Autodesk Inventor part; units mm, degrees
ref_plane "YZ Plane" through (0, 0, 0) normal (1, 0, 0) x (0, 1, 0)
ref_plane "XZ Plane" through (0, 0, 0) normal (0, 1, 0) x (-1, 0, 0)
ref_plane "XY Plane" through (0, 0, 0) normal (0, 0, 1) x (1, 0, 0)
sketch "Sketch1" plane through (0, 0, 0) normal (0, 1, 0) x (-1, 0, 0)
  line L0 (0, -2) -> (0, -29.2)
  line L1 (-2, -31.2) -> (-39, -31.2)
  line L2 (-39, -31.2) -> (-39, -20.2)
  line L3 (-39, -20.2) -> (-37, -20.2)
  line L4 (-37, -20.2) -> (-37, -10.9)
  line L5 (-37, -10.9) -> (-39, -10.9)
  line L6 (-39, -10.9) -> (-39, -2.6)
  line L7 (-39, -2.6) -> (-32.7, -2.6)
  line L8 (-32.7, -2.6) -> (-32.7, 0)
  line L9 (-32.7, 0) -> (-2, 0)
  line L10 (0, -2) -> (-2, 0)
  line L11 (0, -29.2) -> (-2, -31.2)
  point P0 (0, 0)
  point P1 (0, -31.2)
  dimension "d0" = 31.2
  dimension "d1" = 39
  dimension "d2" = 11
  dimension "d3" = 2
  dimension "d4" = 9.3
  dimension "d5" = 8.3
  dimension "d6" = 6.3
  dimension "d7" = 2
  dimension "d8" = 2
  dimension "d9" = 2
  dimension "d10" = 2
extrude "Extrusion1" add sketch "Sketch1" along normal blind 1
sketch "Sketch2" plane through (0, 1, 0) normal (0, 1, 0) x (1, 0, 0)
  line L0 (39, 31.2) -> (2, 31.2)
  line L1 (2, 31.2) -> (0, 29.2)
  line L2 (0, 29.2) -> (0, 2)
  line L3 (0, 2) -> (2, 0)
  line L4 (2, 0) -> (32.7, 0)
  line L5 (32.7, 0) -> (32.7, 2.6)
  line L6 (32.7, 2.6) -> (39, 2.6)
  line L7 (39, 2.6) -> (39, 10.9)
  line L8 (39, 10.9) -> (37, 10.9)
  line L9 (37, 10.9) -> (37, 20.2)
  line L10 (37, 20.2) -> (39, 20.2)
  line L11 (39, 20.2) -> (39, 31.2)
  line L12 (7.2, 7.6) -> (24.7, 7.6)
  line L13 (24.7, 7.6) -> (24.7, 23.1)
  line L14 (24.7, 23.1) -> (7.2, 23.1)
  line L15 (7.2, 23.1) -> (7.2, 7.6)
  line L16 (39, 11.7) -> (33.4, 11.7)
  line L17 (33.4, 11.7) -> (33.4, 19.9)
  line L18 (33.4, 19.9) -> (39, 19.9)
  line L19 (39, 19.9) -> (39, 11.7)
  line L20 (32.7, 2.6) -> (39, 2.6)
  line L21 (33.4, 4.6553) -> (38.4269, 4.6553)
  line L22 (38.4269, 4.6553) -> (38.4269, 2.6)
  line L23 (38.4269, 2.6) -> (33.4, 2.6)
  line L24 (33.4, 2.6) -> (33.4, 4.6553)
  line L25 (34.7176, 2.6) -> (37, 2.6)
  line L26 (37, 2.6) -> (37, 1.3)
  line L27 (37, 1.3) -> (34.7176, 1.3)
  line L28 (34.7176, 1.3) -> (34.7176, 2.6)
  point P0 (0, 0)
  dimension "d13" = 17.5
  dimension "d14" = 15.5
  dimension "d15" = 7.6
  dimension "d16" = 7.2
  dimension "d17" = 5.6
  dimension "d18" = 8.2
  dimension "d19" = 11.7
extrude "Extrusion2" add sketch "Sketch2" along normal blind 2.8 contours L18 L19 L16 L9 | L9 L16 L17 L18 | L24 L21 L22 L6 | L6 L26 L27 L28 | L15 L14 L13 L12
sketch "Sketch3" plane through (0, 1, 0) normal (0, 1, 0) x (1, 0, 0)
  line L0 (2, 0) -> (32.7, 0)
  line L1 (0, 29.2) -> (0, 2)
  point P0 (0, 0)
  point P1 (8, 1.7)
  dimension "d22" = 1.7
  dimension "d23" = 8
hole "Hole1" at (8, 1, -1.7) direction (0, -1, 0) diameter 1 depth 16 tip angle 118
pattern_linear "Rectangular Pattern1" count 10 spacing 2 along (1, 0, 0) of "Hole1"
pattern_linear "Rectangular Pattern2" count 2 spacing 2 along (0, 0, -1) of "Hole1", "Rectangular Pattern1"
ref_plane "Work Plane1" through (2, 0, -15.6) normal (0, 0, 1) x (1, 0, 0)
mirror "Mirror1" [suppressed]
sketch "Sketch4" plane through (2, 0, 0) normal (0, 0, 1) x (1, 0, 0)
  line L0 (5.5, 0) -> (5.5, 1)
  line L1 (6.5, 0) -> (6.5, 1)
  circle A0 centre (6, 2.25) radius 0.5
  line L2 (0, 1) -> (30.7, 1)
  line L3 (5.25, 3) -> (6.75, 3)
  line L4 (6.75, 3) -> (6.75, 1.5)
  line L5 (6.75, 1.5) -> (5.25, 1.5)
  line L6 (5.25, 1.5) -> (5.25, 3)
  line L7 (5.25, 3) -> (6.75, 1.5) construction
  line L8 (6.75, 3) -> (5.25, 1.5) construction
  point P0 (-2, 0)
  dimension "d37" = 1.25
  dimension "d42" = 1.5
  dimension "d43" = 1.5
extrude "Extrusion3" [suppressed]
pattern_linear "Rectangular Pattern3" [suppressed]
mirror "Mirror2" [suppressed]
properties part number "00_ESP32_Mini"
Can you work these out from the model? Positions are in its coordinate system, mm. A direction names the side the tool comes from. Give positions to 0.01 mm unless a question says otherwise; leave off trailing zeros. Loops run counter-clockwise (first coordinate to the right, second up) from the corner with the lowest first, then second, coordinate; pieces in that order, holes last. Notation, with made-up numbers: M 56.5,-20 L 90.5,-20 A17 cw 90.5,-2 Z; hole C 51,28 d10. An arc over 180 degrees is marked long. Use one line per item in the form item = value. Start each with the question number.
(1) I want a section at D-D, the plane x = 34. Write out the boundary of the cut face in (y, z), and give its area (3 significant figures).
(2) I want a section at C-C, the plane z = -10. Write out the boundary of the cut face in (x, y), and give its area (3 significant figures).
(3) I want a section at A-A, the plane y = 2.7. Write out the boundary of the cut face in (x, z).
(4) I'm going to push flat-ended pins straight in: P1, Ø1.9, axis at x = 36.5, y = 2, coming from the +Z side; P2, Ø2, axis at x = 14, y = 2.5, coming from the +Z side; P3, Ø0.5, axis at y = 0.5, z = -1, coming from the +X side. Where does each tip first touch, or does it pass through?
(5) I want a section at B-B, the plane x = 14. Write out the boundary of the cut face in (y, z).
(6) On a 3-axis mill with a long thin cutter (end or side, diameter ignored), from which of +Z, -Z, +X, -X, +Y, -Y can I reach the whole of each face in a straight line? I mean faces 1 (the flat face through (38.427, 2, -4)), 2 (the cylindrical face through (17.504, 0.493, -1.765)), 3 (the flat face through (38, 1, -16)), 4 (the flat face through (24.7, 2, -15)), 5 (the flat face through (16, 2, -23.1)). Say none if no direction works.
(7) Please list where these lines run through material, in increasing order: line 1 (Z direction, x = 12, y = 0.6); line 2 (Z direction, x = 34, y = 3.3); line 3 (X direction, y = 1.7, z = -12).
(8) Thinking about a two-plate mould opening in Z: for faces 6 (the flat face through (16, 3.8, -15)), 7 (the cylindrical face through (13.504, 0.493, -1.765)), 8 (the flat face through (20.2, 0.5, -31.2)), 9 (the cylindrical face through (13.504, 0.493, -3.765)), which applies, released by +Z, released by -Z, zero draft, split by the parting line, or undercut?
Worked out:
q1.outline = M 0,-31.2 L 1,-31.2 L 1,-19.9 L 3.8,-19.9 L 3.8,-11.7 L 1,-11.7 L 1,-4.66 L 3.8,-4.66 L 3.8,-2.6 L 0,-2.6 Z
q1.area = 57.3 mm²
q2.outline = M 0,0 L 39,0 L 39,1 L 24.7,1 L 24.7,3.8 L 7.2,3.8 L 7.2,1 L 0,1 Z
q2.area = 88.0 mm²
q3.outline = M 7.2,-23.1 L 24.7,-23.1 L 24.7,-7.6 L 7.2,-7.6 Z; M 33.4,-19.9 L 39,-19.9 L 39,-11.7 L 33.4,-11.7 Z; M 33.4,-4.66 L 38.43,-4.66 L 38.43,-2.6 L 37,-2.6 L 37,-1.3 L 34.72,-1.3 L 34.72,-2.6 L 33.4,-2.6 Z
q4.P1 = -1.3
q4.P2 = -7.6
q4.P3 = 32.7
q5.outline = M 0,-31.2 L 1,-31.2 L 1,-23.1 L 3.8,-23.1 L 3.8,-7.6 L 1,-7.6 L 1,-4.2 L 0,-4.2 Z; M 0,-3.2 L 1,-3.2 L 1,-2.2 L 0,-2.2 Z; M 0,-1.2 L 1,-1.2 L 1,0 L 0,0 Z
q6.face_1 = +Z, +X, +Y
q6.face_2 = +Y, -Y
q6.face_3 = +X, -Y
q6.face_4 = +Z, -Z, +Y
q6.face_5 = -Z, +X, -X, +Y
q7.line_1 = -31.2 to -4.2, -3.2 to -2.2, -1.2 to 0
q7.line_2 = -19.9 to -11.7, -4.66 to -2.6
q7.line_3 = 7.2 to 24.7, 33.4 to 39
q8.face_6 = zero draft
q8.face_7 = undercut
q8.face_8 = released by -Z
q8.face_9 = undercut
